from build123d import *

# Parameters (mm, degrees)
DODANIE_WYCI_GNI_CIE1_DEPTH = 5
WYTNIJ_WYCI_GNI_CIE1_DEPTH  = 3
ZAOKR_GLENIE3_R             = 3
WYTNIJ_WYCI_GNI_CIE3_DEPTH  = 108.951175455
ZAOKR_GLENIE4_R             = 3


with BuildPart() as part:
    # Szkic1 → Dodanie-wyci_gni_cie1 (new body)
    with BuildSketch(Plane.XY):
        with BuildLine():
            Line((0, 0), (-90, 0))
            Line((-90, 0), (-89.375, -5))
            Line((-89.375, -5), (-85, -5))
            ThreePointArc((-85, -5), (-81.464466094, -6.464466094), (-80, -10))
            ThreePointArc((-80, -10), (-81.464466094, -13.535533906), (-85, -15))
            Line((-85, -15), (-88.125, -15))
            Line((-88.125, -15), (-82.5, -60))
            Line((-82.5, -60), (0, -60))
            Line((0, -60), (0, 0))
        make_face()
        with BuildLine():
            Line((-85, -5), (-89.375, -5))
            Line((-89.375, -5), (-89.106551139, -7.147590888))
            ThreePointArc((-89.106551139, -7.147590888), (-87.317105354, -5.569308995), (-85, -5))
        make_face()
        with BuildLine():
            ThreePointArc((-80, -10), (-81.464466094, -6.464466094), (-85, -5))
            Line((-85, -5), (-85, -7.75))
            ThreePointArc((-85, -7.75), (-83.409009742, -8.409009742), (-82.75, -10))
            ThreePointArc((-82.75, -10), (-83.409009742, -11.590990258), (-85, -12.25))
            Line((-85, -12.25), (-85, -15))
            ThreePointArc((-85, -15), (-81.464466094, -13.535533906), (-80, -10))
        make_face()
        with BuildLine():
            ThreePointArc((-85, -5), (-87.317105354, -5.569308995), (-89.106551139, -7.147590888))
            Line((-89.106551139, -7.147590888), (-88.278064246, -13.775486035))
            ThreePointArc((-88.278064246, -13.775486035), (-86.749652798, -14.68387821), (-85, -15))
            Line((-85, -15), (-85, -12.25))
            ThreePointArc((-85, -12.25), (-87.25, -10), (-85, -7.75))
            Line((-85, -7.75), (-85, -5))
        make_face()
        with BuildLine():
            ThreePointArc((-85, -15), (-86.749652798, -14.68387821), (-88.278064246, -13.775486035))
            Line((-88.278064246, -13.775486035), (-88.125, -15))
            Line((-88.125, -15), (-85, -15))
        make_face()
    extrude(amount=DODANIE_WYCI_GNI_CIE1_DEPTH)

    # Szkic1_3 → Wytnij-wyci_gni_cie1 (cut)
    with BuildSketch(Plane.XY):
        with BuildLine():
            ThreePointArc((-80, -10), (-81.464466094, -6.464466094), (-85, -5))
            Line((-85, -5), (-85, -7.75))
            ThreePointArc((-85, -7.75), (-83.409009742, -8.409009742), (-82.75, -10))
            ThreePointArc((-82.75, -10), (-83.409009742, -11.590990258), (-85, -12.25))
            Line((-85, -12.25), (-85, -15))
            ThreePointArc((-85, -15), (-81.464466094, -13.535533906), (-80, -10))
        make_face()
        with BuildLine():
            ThreePointArc((-85, -5), (-87.317105354, -5.569308995), (-89.106551139, -7.147590888))
            Line((-89.106551139, -7.147590888), (-88.278064246, -13.775486035))
            ThreePointArc((-88.278064246, -13.775486035), (-86.749652798, -14.68387821), (-85, -15))
            Line((-85, -15), (-85, -12.25))
            ThreePointArc((-85, -12.25), (-87.25, -10), (-85, -7.75))
            Line((-85, -7.75), (-85, -5))
        make_face()
        with BuildLine():
            Line((-85, -5), (-89.375, -5))
            Line((-89.375, -5), (-89.106551139, -7.147590888))
            ThreePointArc((-89.106551139, -7.147590888), (-87.317105354, -5.569308995), (-85, -5))
        make_face()
        with BuildLine():
            ThreePointArc((-85, -15), (-86.749652798, -14.68387821), (-88.278064246, -13.775486035))
            Line((-88.278064246, -13.775486035), (-88.125, -15))
            Line((-88.125, -15), (-85, -15))
        make_face()
    extrude(amount=WYTNIJ_WYCI_GNI_CIE1_DEPTH, mode=Mode.SUBTRACT)

    # Zaokr_glenie3
    zaokr_glenie3_edges = [part.edges().sort_by_distance(p)[0] for p in [
        (-82.5, -60, 2.5),
        (-90, 0, 2.5),
    ]]
    fillet(zaokr_glenie3_edges, radius=ZAOKR_GLENIE3_R)

    # Szkic5 → Wytnij-wyci_gni_cie3 (cut, through all)
    with BuildSketch(Plane(origin=(0, 0, 0), x_dir=(-1, 0, 0), z_dir=(0, 0, -1))):
        with BuildLine():
            Line((5, -55), (78.086088907, -55))
            Line((78.086088907, -55), (82.500757178, -19.682653836))
            ThreePointArc((82.500757178, -19.682653836), (75.778900637, -13.869279847), (76.339745962, -5))
            Line((76.339745962, -5), (5, -5))
            Line((5, -5), (5, -55))
        make_face()
    extrude(amount=-WYTNIJ_WYCI_GNI_CIE3_DEPTH, mode=Mode.SUBTRACT)

    # Zaokr_glenie4
    zaokr_glenie4_edges = [part.edges().sort_by_distance(p)[0] for p in [
        (-5, -5, 2.5),
        (-76.339745962, -5, 2.5),
        (-82.500757178, -19.682653836, 2.5),
        (-78.086088907, -55, 2.5),
        (-5, -55, 2.5),
    ]]
    fillet(zaokr_glenie4_edges, radius=ZAOKR_GLENIE4_R)

    # Lustro5: part across plane


with BuildPart() as part_1:
    add(part.part)
    add(part.part.mirror(Plane(origin=(0, 0, 0), x_dir=(0, 0, 1), z_dir=(1, 0, 0))))


solid = part_1.part
Design review of the part built by this model. Coordinates are the model's own, in mm. A direction names the side the tool comes from. Give positions to 0.01 mm unless a question says otherwise; leave off trailing zeros. Write each loop counter-clockwise with the first axis right and the second up, starting at its lowest first coordinate (ties: lowest second). Pieces come first, ordered by that corner, then holes. Notation, with made-up numbers: M 81.25,11 L 115.25,11 A27 cw 115.25,39 Z; hole C 9,75 d9. An arc over 180 degrees is marked long. Answer as a JSON object with one key per item and string values. Group by question number.
1) We need section C-C (z = 4.05). Count the separate pieces of the cut face and the enclosed holes in it, and give its area (3 significant figures).
2) Clearance check with flat-ended pins moving along their axes: pin 1 Ø1.5 at (y, z) = (-51.5, 4) entering from -X; pin 2 Ø1 at (y, z) = (-18, 3.5) entering from -X; pin 3 Ø1.5 at (y, z) = (-15.5, 1.5) entering from -X (3 decimals). State where each tip first meets the part, or that it passes through.
3) We need section B-B (y = -31). Give the boundary of the cut face in (x, z) (3 decimals), and give its area (3 significant figures).
4) Tool access review of faces 1 (the face through (-76.163, -14.681, 2.465)), 2 (the face through (-87, -5, 1)), 3 (the face through (87, -5, 1)): name each direction out of +Z, -Z, +X, -X, +Y, -Y from which nothing blocks a thin tool from reaching the whole face with its end or side.
5) For line 1 along Y through (x, z) = (18, 3.2); line 2 along X through (y, z) = (-15.5, 4.75); line 3 along X through (y, z) = (-44, 3.95), list the stretches that pass through material, from the lowest coordinate up.
6) We need section A-A (x = -40). Give the boundary of the cut face in (y, z).
Answer key:
{
 "1": {"separate pieces": "1", "enclosed holes": "4", "area": "2,910 mm²"},
 "2": {"pin 1": "stops at x = -83.66", "pin 2": "stops at x = -87.81", "pin 3": "stops at x = -88.125"},
 "3": {"outline": "M -86.125,0 L -81.086,0 L -81.086,5 L -86.125,5 Z; M -5,0 L 5,0 L 5,5 L -5,5 Z; M 81.086,0 L 86.125,0 L 86.125,5 L 81.086,5 Z", "area": "100 mm²"},
 "4": {"face 1": "+Z, -Z", "face 2": "-Z, -X", "face 3": "-Z, +X"},
 "5": {"line 1": "y = -60 to -55, -5 to 0", "line 2": "x = -88.06 to -76.65, -5 to 5, 76.65 to 88.06", "line 3": "x = -84.5 to -79.46, -5 to 5, 79.46 to 84.5"},
 "6": {"outline": "M -60,0 L -55,0 L -55,5 L -60,5 Z; M -5,0 L 0,0 L 0,5 L -5,5 Z"}
}
